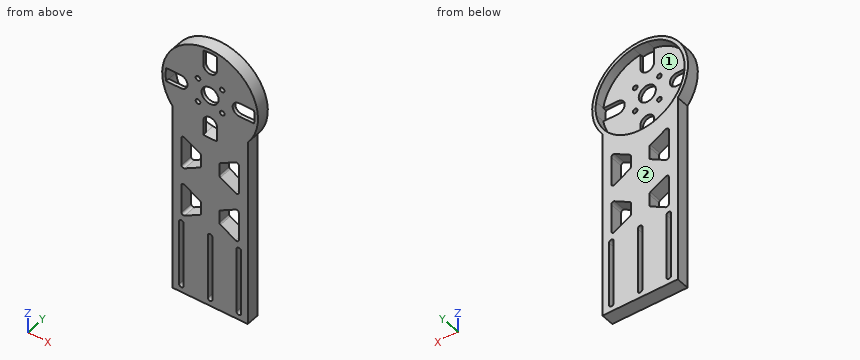
```python
from build123d import *

# Parameters (mm, degrees)
BOSS_EXTRUDE1_OUTLINE_R = 6.25
BOSS_EXTRUDE1_DEPTH     = 9.525
CUT_EXTRUDE1_START      = -7
SKETCH3_R               = 32.5
CUT_EXTRUDE1_DEPTH      = 7
M3_CLEARANCE_HOLE1_D    = 3.4


# Read off the part's stored shape, not the designer's step: Boss-Extrude1
with BuildPart() as part:
    # Boss-Extrude1 outline → Boss-Extrude1 (new body)
    with BuildSketch(Plane(origin=(0, 0, 0), x_dir=(1, 0, 0), z_dir=(0, 1, 0))):
        with BuildLine():
            Line((-27.5, 160), (-27.5, 21.650635095))
            ThreePointArc((-27.5, 21.650635095), (0, -35), (27.5, 21.650635095))
            Line((27.5, 21.650635095), (27.5, 160))
            Line((27.5, 160), (-27.5, 160))
        make_face()
        with BuildLine():
            Line((-21.67, -5), (-32.113081447, -5))
            ThreePointArc((-32.113081447, -5), (-32.5, 0), (-32.113081447, 5))
            Line((-32.113081447, 5), (-21.67, 5))
            ThreePointArc((-21.67, 5), (-21.6199975, 4.999749969), (-21.57, 4.9989999))
            ThreePointArc((-21.57, 4.9989999), (-16.47, 0), (-21.57, -4.9989999))
            ThreePointArc((-21.57, -4.9989999), (-21.6199975, -4.999749969), (-21.67, -5))
        make_face(mode=Mode.SUBTRACT)
        with BuildLine():
            Line((-21, 42.707149814), (-21, 63.292850186))
            ThreePointArc((-21, 63.292850186), (-20.2155368, 64.662261792), (-18.637432255, 64.678283779))
            Line((-18.637432255, 64.678283779), (-7.512432255, 58.454507556))
            ThreePointArc((-7.512432255, 58.454507556), (-6.918088394, 57.872110763), (-6.7, 57.069073962))
            Line((-6.7, 57.069073962), (-6.7, 48.930926038))
            ThreePointArc((-6.7, 48.930926038), (-6.918088394, 48.127889237), (-7.512432255, 47.545492444))
            Line((-7.512432255, 47.545492444), (-18.637432255, 41.321716221))
            ThreePointArc((-18.637432255, 41.321716221), (-20.2155368, 41.337738208), (-21, 42.707149814))
        make_face(mode=Mode.SUBTRACT)
        with BuildLine():
            Line((5, -21.872218084), (5, -32.113081447))
            ThreePointArc((5, -32.113081447), (0, -32.5), (-5, -32.113081447))
            Line((-5, -32.113081447), (-5, -21.872218084))
            ThreePointArc((-5, -21.872218084), (-4.998988367, -21.771643214), (-4.995953878, -21.671109042))
            ThreePointArc((-4.995953878, -21.671109042), (0, -16.47), (4.995953878, -21.671109042))
            ThreePointArc((4.995953878, -21.671109042), (4.998988367, -21.771643214), (5, -21.872218084))
        make_face(mode=Mode.SUBTRACT)
        Circle(BOSS_EXTRUDE1_OUTLINE_R, mode=Mode.SUBTRACT)
        with BuildLine():
            Line((21.67, 5), (32.113081447, 5))
            ThreePointArc((32.113081447, 5), (32.5, 0), (32.113081447, -5))
            Line((32.113081447, -5), (21.67, -5))
            ThreePointArc((21.67, -5), (21.6199975, -4.999749969), (21.57, -4.9989999))
            ThreePointArc((21.57, -4.9989999), (16.47, 0), (21.57, 4.9989999))
            ThreePointArc((21.57, 4.9989999), (21.6199975, 4.999749969), (21.67, 5))
        make_face(mode=Mode.SUBTRACT)
        with BuildLine():
            Line((-5, 21.466517846), (-5, 32.113081447))
            ThreePointArc((-5, 32.113081447), (0, 32.5), (5, 32.113081447))
            Line((5, 32.113081447), (5, 21.466517846))
            ThreePointArc((5, 21.466517846), (0, 16.466517846), (-5, 21.466517846))
        make_face(mode=Mode.SUBTRACT)
        with BuildLine():
            ThreePointArc((7.512432255, 47.545492444), (6.918088394, 48.127889237), (6.7, 48.930926038))
            Line((6.7, 48.930926038), (6.7, 57.069073962))
            ThreePointArc((6.7, 57.069073962), (6.918088394, 57.872110763), (7.512432255, 58.454507556))
            Line((7.512432255, 58.454507556), (18.637432255, 64.678283779))
            ThreePointArc((18.637432255, 64.678283779), (20.2155368, 64.662261792), (21, 63.292850186))
            Line((21, 63.292850186), (21, 42.707149814))
            ThreePointArc((21, 42.707149814), (20.2155368, 41.337738208), (18.637432255, 41.321716221))
            Line((18.637432255, 41.321716221), (7.512432255, 47.545492444))
        make_face(mode=Mode.SUBTRACT)
        with BuildLine():
            Line((-21, 78.707149814), (-21, 99.292850186))
            ThreePointArc((-21, 99.292850186), (-20.2155368, 100.662261792), (-18.637432255, 100.678283779))
            Line((-18.637432255, 100.678283779), (-7.512432255, 94.454507556))
            ThreePointArc((-7.512432255, 94.454507556), (-6.918088394, 93.872110763), (-6.7, 93.069073962))
            Line((-6.7, 93.069073962), (-6.7, 84.930926038))
            ThreePointArc((-6.7, 84.930926038), (-6.918088394, 84.127889237), (-7.512432255, 83.545492444))
            Line((-7.512432255, 83.545492444), (-18.637432255, 77.321716221))
            ThreePointArc((-18.637432255, 77.321716221), (-20.2155368, 77.337738208), (-21, 78.707149814))
        make_face(mode=Mode.SUBTRACT)
        with BuildLine():
            Line((-19.3, 154.596553922), (-19.3, 107))
            ThreePointArc((-19.3, 107), (-21, 105.3), (-22.7, 107))
            Line((-22.7, 107), (-22.7, 154.596553922))
            ThreePointArc((-22.7, 154.596553922), (-21, 156.296553922), (-19.3, 154.596553922))
        make_face(mode=Mode.SUBTRACT)
        with BuildLine():
            ThreePointArc((18.637432255, 100.678283779), (20.2155368, 100.662261792), (21, 99.292850186))
            Line((21, 99.292850186), (21, 78.707149814))
            ThreePointArc((21, 78.707149814), (20.2155368, 77.337738208), (18.637432255, 77.321716221))
            Line((18.637432255, 77.321716221), (7.512432255, 83.545492444))
            ThreePointArc((7.512432255, 83.545492444), (6.918088394, 84.127889237), (6.7, 84.930926038))
            Line((6.7, 84.930926038), (6.7, 93.069073962))
            ThreePointArc((6.7, 93.069073962), (6.918088394, 93.872110763), (7.512432255, 94.454507556))
            Line((7.512432255, 94.454507556), (18.637432255, 100.678283779))
        make_face(mode=Mode.SUBTRACT)
        with BuildLine():
            Line((1.7, 154.596553922), (1.7, 107))
            ThreePointArc((1.7, 107), (0, 105.3), (-1.7, 107))
            Line((-1.7, 107), (-1.7, 154.596553922))
            ThreePointArc((-1.7, 154.596553922), (0, 156.296553922), (1.7, 154.596553922))
        make_face(mode=Mode.SUBTRACT)
        with BuildLine():
            Line((22.7, 154.596553922), (22.7, 107))
            ThreePointArc((22.7, 107), (21, 105.3), (19.3, 107))
            Line((19.3, 107), (19.3, 154.596553922))
            ThreePointArc((19.3, 154.596553922), (21, 156.296553922), (22.7, 154.596553922))
        make_face(mode=Mode.SUBTRACT)
    extrude(amount=BOSS_EXTRUDE1_DEPTH)

    # Sketch3 → Cut-Extrude1 (cut)
    with BuildSketch(Plane(origin=(0, 9.525, 0), x_dir=(1, 0, 0), z_dir=(0, 1, 0)).offset(CUT_EXTRUDE1_START)):
        with Locations(Location((0, 0, 0), (0, 0, 81.150116902))):
            Circle(SKETCH3_R)
    extrude(amount=CUT_EXTRUDE1_DEPTH, mode=Mode.SUBTRACT)

    # M3 Clearance Hole1 (through all)
    with Locations(Plane(origin=(0, 2.525, 0), x_dir=(1, 0, 0), z_dir=(0, 1, 0))):
        with Locations((8.838834765, 8.838834765), (-8.838834765, -8.838834765), (-8.838834765, 8.838834765), (8.838834765, -8.838834765)):
            Hole(M3_CLEARANCE_HOLE1_D / 2)


solid = part.part
```
Here's how the part is built. I have some questions about the finished solid (model axes, mm). Face numbers are marked on the shaded views. Coordinates: 2 decimals unless noted, no trailing zeros. Order: outer loops, then holes, each group sorted by start corner. A loop starts at its lowest first (then second) coordinate and runs counter-clockwise, first axis right, second up. Notation, with made-up numbers: (32.5, 61) - (77.5, 61) arc R22 cw to (77.5, 92) - close; hole circle Ø11 at (16, 3). An arc over 180 degrees is marked (long way). One line per question, with ' | ' between items.
(1) Suppose I cut it at C-C on x = 0. List the corners of the cut face in (y, z) for me (3 decimals), and give its area (3 significant figures).
Report:
outline: (0, -160) - (9.525, -160) - (9.525, -156.297) - (0, -156.297) - close; (0, -105.3) - (9.525, -105.3) - (9.525, -32.5) - (0, -32.5) - close; (0, -16.467) - (2.525, -16.467) - (2.525, -6.25) - (0, -6.25) - close; (0, 6.25) - (2.525, 6.25) - (2.525, 16.47) - (0, 16.47) - close; (0, 32.5) - (9.525, 32.5) - (9.525, 35) - (0, 35) - close | area: 804 mm2
(2) Suppose I cut it at D-D on x = 29.5. List the corners of the cut face in (y, z) for me (3 decimals), and give its area (3 significant figures).
Report:
outline: (0, -18.835) - (9.525, -18.835) - (9.525, -13.638) - (2.525, -13.638) - (2.525, -5) - (0, -5) - close; (0, 5) - (2.525, 5) - (2.525, 13.638) - (9.525, 13.638) - (9.525, 18.835) - (0, 18.835) - close | area: 143 mm2
(3) Suppose I cut it at B-B on x = -13. List the corners of the cut face in (y, z) for me (3 decimals), and give its area (3 significant figures).
Report:
outline: (0, -160) - (9.525, -160) - (9.525, -97.524) - (0, -97.524) - close; (0, -80.476) - (9.525, -80.476) - (9.525, -61.524) - (0, -61.524) - close; (0, -44.476) - (9.525, -44.476) - (9.525, -29.787) - (2.525, -29.787) - (2.525, 29.787) - (9.525, 29.787) - (9.525, 32.496) - (0, 32.496) - close | area: 1,090 mm2
(4) If we mould it in two halves opening along Z, with no side actions, what happens to the marked faces 1 and 2? For each: pulls with the +Z half, pulls with the -Z half, needs draft (parallel to the pull), parting line crosses it, or undercut.
Report:
face 1: undercut | face 2: needs draft
(5) If I drill on L1, parallel to Z at x = 0, y = 1.7; L2, parallel to X at y = 7.75, z = -140; L3, parallel to X at y = 1.3, z = 0, over which ranges is the centre line in solid material (lowest first)?
Report:
L1: z = -160 to -156.3, -105.3 to -32.5, -16.47 to -6.25, 6.25 to 16.47, 32.5 to 35 | L2: x = -27.5 to -22.7, -19.3 to -1.7, 1.7 to 19.3, 22.7 to 27.5 | L3: x = -35 to -32.5, -16.47 to -6.25, 6.25 to 16.47, 32.5 to 35
(6) Suppose I cut it at A-A on z = 0. List the corners of the cut face in (x, y) for me (3 decimals).
Report:
outline: (-35, 0) - (-32.5, 0) - (-32.5, 9.525) - (-35, 9.525) - close; (-16.47, 0) - (-6.25, 0) - (-6.25, 2.525) - (-16.47, 2.525) - close; (6.25, 0) - (16.47, 0) - (16.47, 2.525) - (6.25, 2.525) - close; (32.5, 0) - (35, 0) - (35, 9.525) - (32.5, 9.525) - close
(7) Will these pins go through, and if not, where does the flat tip stop? pin 1 (2 mm diameter, centred on y = 1.5, z = -29, fed in from +X); pin 2 (1 mm diameter, centred on x = 2, y = 2, fed in from +Z); pin 3 (3 mm diameter, centred on y = 5.5, z = -139.5, fed in from -X).
Report:
pin 1: stops at x = 27.5 | pin 2: stops at z = 34.97 | pin 3: stops at x = -27.5
